For this review, take the finished solid that the model builds, in its own axes (mm). A direction names the side the tool comes from. Round coordinates to 2 decimals unless told otherwise and drop trailing zeros. Order: outer loops, then holes, each group sorted by start corner. A loop starts at its lowest first (then second) coordinate and runs counter-clockwise, first axis right, second up. Notation, with made-up numbers: (31, 5) -> (64, 5) arc R38 cw to (64, 44) -> close; hole circle Ø6 at (11, 85). An arc over 180 degrees is marked (long way). Put each result on its own line as item: value. Start each with the question number.
```python
from build123d import *

# Parameters (mm, degrees)
F0_W     = 76
F0_H     = 21
F1_DEPTH = 19
F2_W     = 72
F2_H     = 17
F3_DEPTH = 17
F4_R     = 1.5
F5_DEPTH = 19.001
F6_R     = 1.25
F7_DEPTH = 2
F9_DEPTH = 2


with BuildPart() as f1:
    # F0 (on Top) → F1 (new body)
    with BuildSketch(Plane.XY):
        Rectangle(F0_W, F0_H)
    extrude(amount=F1_DEPTH)

    # F2 (on face) → F3 (cut)
    with BuildSketch(Plane.XY.offset(19)):
        Rectangle(F2_W, F2_H)
    extrude(amount=-F3_DEPTH, mode=Mode.SUBTRACT)

    # F4 (on face) → F5 (cut, through all)
    with BuildSketch(Plane(origin=(0, 0, 0), x_dir=(1, 0, 0), z_dir=(0, 0, -1))):
        Circle(F4_R)
    extrude(amount=-F5_DEPTH, mode=Mode.SUBTRACT)

    # F6 (on face) → F7 (cut)
    with BuildSketch(Plane(origin=(-38, 0, 0), x_dir=(0, -1, 0), z_dir=(-1, 0, 0))):
        with Locations((7.5, 2)):
            Circle(F6_R)
    extrude(amount=-F7_DEPTH, mode=Mode.SUBTRACT)

    # F8 (on face) → F9 (cut)
    with BuildSketch(Plane.YZ.offset(38)):
        with BuildLine():
            ThreePointArc((7.5, 0.75), (8.383883, 1.116117), (8.75, 2))
            Line((8.75, 2), (7.5, 2))
            Line((7.5, 2), (7.5, 0.75))
        make_face()
        with BuildLine():
            Line((7.5, 2), (8.75, 2))
            ThreePointArc((8.75, 2), (6.616117, 2.883883), (7.5, 0.75))
            Line((7.5, 0.75), (7.5, 2))
        make_face()
    extrude(amount=-F9_DEPTH, mode=Mode.SUBTRACT)


solid = f1.part
```
Item 1: Insertion check: pin 1 Ø3.5 at (x, y) = (0, 0) entering from +Z; pin 2 Ø1.5 at (y, z) = (-7.5, 2) entering from -X; pin 3 Ø0.6 at (y, z) = (7.5, 2) entering from +X. Each pin has a flat end and moves straight along its axis. Give the tip position at first contact, or say it passes through.
Item 2: For L1, parallel to Y at x = 2, z = 8.5; L2, parallel to X at y = -6, z = 18.25; L3, parallel to Z at x = -37.5, y = -7.5, list the stretches that pass through material, from the lowest coordinate up.
Item 3: Consider section C-C, the plane z = 16.5. Write out the cut boundary in (x, y).
Item 4: Tool access review of faces 1 (the face through (38, 0, 9)), 2 (the face through (-37.01, -6.25, 2.05)), 3 (the face through (-36, 0, 11)): name each direction out of +Z, -Z, +X, -X, +Y, -Y from which nothing blocks a thin tool from reaching the whole face with its end or side.
Item 5: Consider section D-D, the plane x = 26. Write out the cut boundary in (y, z).
Item 6: Mouldability with a two-part tool opening along Z and no side actions: class faces 4 (the face through (36, 7.5, 1.5)), 5 (the face through (-1, 2, 0)), 6 (the face through (-1, 8.5, 11)) as +Z half, -Z half, draft (parallel to the pull), parting line (faces both ways), or undercut.
Item 7: Consider section B-B, the plane x = 0. Write out the cut boundary in (y, z), plus the area to 3 significant figures.
Item 8: Consider section A-A, the plane y = -7.5. Write out the cut boundary in (x, z).
Evaluation:
1. pin 1: stops at z = 2
1. pin 2: stops at x = -36
1. pin 3: stops at x = 36
2. L1: y = -10.5 to -8.5, 8.5 to 10.5
2. L2: x = -38 to -36, 36 to 38
2. L3: z = 0 to 0.75, 3.25 to 19
3. outline: (-38, -10.5) -> (38, -10.5) -> (38, 10.5) -> (-38, 10.5) -> close; hole (-36, -8.5) -> (36, -8.5) -> (36, 8.5) -> (-36, 8.5) -> close
4. face 1: +Z, -Z, +X, +Y, -Y
4. face 2: -X
4. face 3: +Z
5. outline: (-10.5, 0) -> (10.5, 0) -> (10.5, 19) -> (8.5, 19) -> (8.5, 2) -> (-8.5, 2) -> (-8.5, 19) -> (-10.5, 19) -> close
6. face 4: undercut
6. face 5: -Z half
6. face 6: draft
7. outline: (-10.5, 0) -> (-1.5, 0) -> (-1.5, 2) -> (-8.5, 2) -> (-8.5, 19) -> (-10.5, 19) -> close; (1.5, 0) -> (10.5, 0) -> (10.5, 19) -> (8.5, 19) -> (8.5, 2) -> (1.5, 2) -> close
7. area: 104 mm^2
8. outline: (-38, 0) -> (38, 0) -> (38, 19) -> (36, 19) -> (36, 2) -> (-36, 2) -> (-36, 0.75) -> (-38, 0.75) -> close; (-38, 3.25) -> (-36, 3.25) -> (-36, 19) -> (-38, 19) -> close
